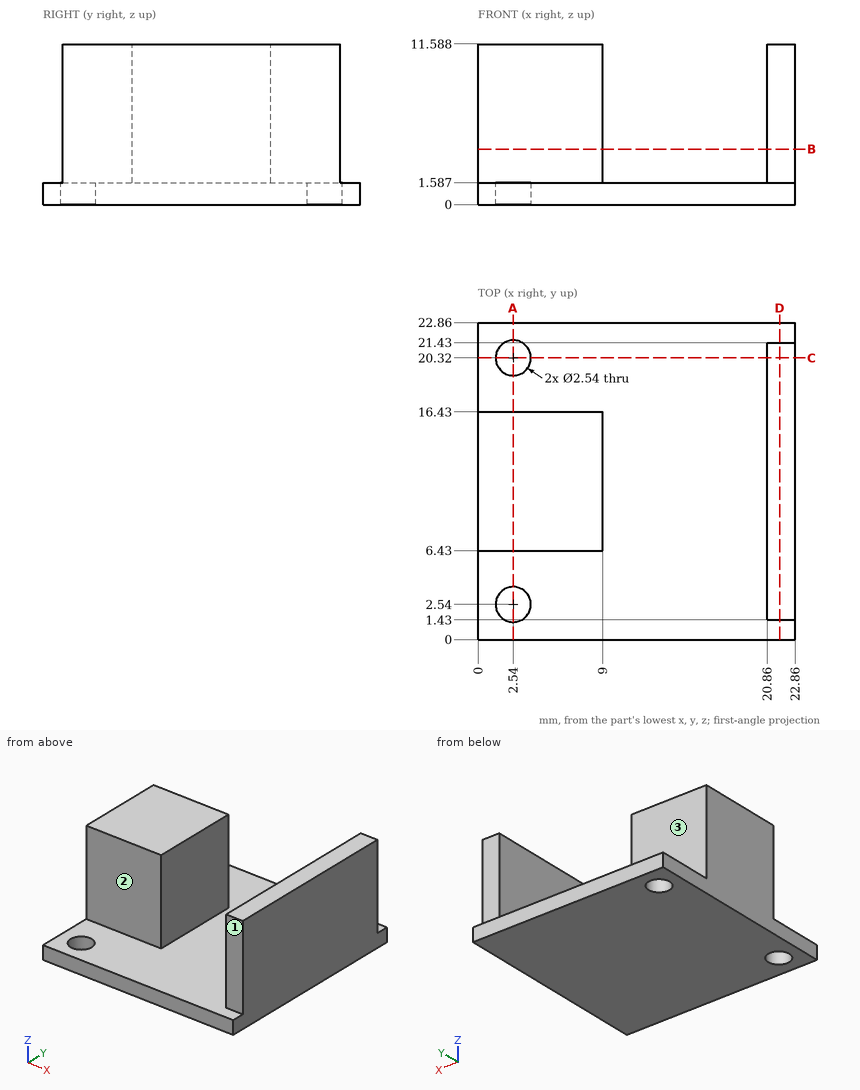
Study the drawing (mm; zero at the part's minimum x, y, z) and answer. A direction names the side the tool comes from. Round coordinates to 2 decimals unless told otherwise and drop trailing zeros. Write each loop counter-clockwise with the first axis right and the second up, starting at its lowest first coordinate (ties: lowest second). Pieces come first, ordered by that corner, then holes.
Q1. Find section C-C on y = 20.32. Determine the outline of the cut face in (x, z).
Values:
outline: (0, 0) - (1.27, 0) - (1.27, 1.59) - (0, 1.59) - close; (3.81, 0) - (22.86, 0) - (22.86, 11.59) - (20.86, 11.59) - (20.86, 1.59) - (3.81, 1.59) - close
Q2. Straight lines are drawn through the part: line 1 (Y direction, x = 2.54, z = 1.1); line 2 (X direction, y = 7.5, z = 9.25); line 3 (Z direction, x = 7, y = 21.5). For each, find the intervals that lie inside material, in ascending order.
Values:
line 1: y = 0 to 1.27, 3.81 to 19.05, 21.59 to 22.86
line 2: x = 0 to 9, 20.86 to 22.86
line 3: z = 0 to 1.59
Q3. Find section D-D on x = 21.75. Determine the outline of the cut face in (y, z).
Values:
outline: (0, 0) - (22.86, 0) - (22.86, 1.59) - (21.43, 1.59) - (21.43, 11.59) - (1.43, 11.59) - (1.43, 1.59) - (0, 1.59) - close
Q4. Find section B-B on z = 4. Determine the outline of the cut face in (x, y), and give its area (3 significant figures).
Values:
outline: (0, 6.43) - (9, 6.43) - (9, 16.43) - (0, 16.43) - close; (20.86, 1.43) - (22.86, 1.43) - (22.86, 21.43) - (20.86, 21.43) - close
area: 130 mm2
Q5. A tool of negligible diameter and unlimited length cuts with its end or side. For the marked faces 1, 2 and 3, from which of +Z, -Z, +X, -X, +Y, -Y can it reach the whole face along a straight path? Write none if from no direction.
Values:
face 1: +Z, +X, -X, -Y
face 2: +Z, -X, -Y
face 3: +Z, -X, +Y
Q6. Find section A-A on x = 2.54. Determine the outline of the cut face in (y, z), and give its area (3 significant figures).
Values:
outline: (0, 0) - (1.27, 0) - (1.27, 1.59) - (0, 1.59) - close; (3.81, 0) - (19.05, 0) - (19.05, 1.59) - (16.43, 1.59) - (16.43, 11.59) - (6.43, 11.59) - (6.43, 1.59) - (3.81, 1.59) - close; (21.59, 0) - (22.86, 0) - (22.86, 1.59) - (21.59, 1.59) - close
area: 128 mm2
Q7. Flat-ended cylindrical pins translate along their axes: P1, Ø2, axis at x = 8, z = 8.5, coming from the -Y side; P2, Ø1.6, axis at x = 22, z = 8, coming from the +Y side; P3, Ø4, axis at x = 2.54, y = 2.54, coming from the +Z side. Find the tip coordinate at first contact, or state that the pin passes through.
Values:
P1: stops at y = 6.43
P2: stops at y = 21.43
P3: stops at z = 1.59
